```python
from build123d import *

# Parameters (mm, degrees)
SKETCH1_R           = 2.9718
SKETCH1_W           = 47.1424
SKETCH1_H           = 22.225
SKETCH1_R_2         = 2.4892
BOSS_EXTRUDE1_DEPTH = 3.175
SKETCH2_W           = 85.2424
SKETCH2_H           = 3.175
BOSS_EXTRUDE2_DEPTH = 3.175


with BuildPart() as part:
    # Sketch1 → Boss-Extrude1 (new body)
    with BuildSketch(Plane.XY):
        Polygon((37.4777, 9.5377), (24.7777, 9.5377), (-35.0647, 9.5377), (-47.7647, 9.5377), (-47.7647, -25.3873), (-35.0647, -25.3873), (12.0777, -25.3873), (24.7777, -25.3873), (37.4777, -25.3873), align=None)
        with Locations((-32.941818083, -7.9248)):
            Circle(SKETCH1_R, mode=Mode.SUBTRACT)
        with Locations((-5.1435, -7.9248)):
            Rectangle(SKETCH1_W, SKETCH1_H, mode=Mode.SUBTRACT)
        with Locations((23.471581917, -7.9248)):
            Circle(SKETCH1_R, mode=Mode.SUBTRACT)
        Polygon((37.4777, -41.2623), (37.4777, -25.3873), (24.7777, -25.3873), (12.0777, -25.3873), (12.0777, -41.2623), align=None)
        with Locations((23.471581917, -33.3248)):
            Circle(SKETCH1_R_2, mode=Mode.SUBTRACT)
    extrude(amount=BOSS_EXTRUDE1_DEPTH)

    # Sketch2 → Boss-Extrude2 (add)
    with BuildSketch(Plane(origin=(0, 0, 0), x_dir=(-1, 0, 0), z_dir=(0, 0, -1))):
        with Locations((5.1435, 7.9502)):
            Rectangle(SKETCH2_W, SKETCH2_H)
    extrude(amount=BOSS_EXTRUDE2_DEPTH)


solid = part.part
```
Geometry check sheet. Reference: the model listing, model coordinates, mm. A direction names the side the tool comes from. Give positions to 0.01 mm unless a question says otherwise; leave off trailing zeros. Order: outer loops, then holes, each group sorted by start corner. A loop starts at its lowest first (then second) coordinate and runs counter-clockwise, first axis right, second up. Notation, with made-up numbers: (-35, -35.75) -> (18, -35.75) arc R23 ccw to (18, -19.75) -> close; hole circle Ø1 at (48, 59). An arc over 180 degrees is marked (long way). Write each question's results on one line, items separated by ' | '. Start each with the question number.
(1) Sectioned sample at D-D (y = -7). Enter the section's corners in (x, z) (3 decimals).
(2) Scan lines: line 1 (X direction, y = -8, z = 2); line 2 (Y direction, x = 18, z = 2); line 3 (Y direction, x = -10, z = -1.5). Record each from-to range of solid material in increasing order.
(3) Access from +Z, -Z, +X, -X, +Y, -Y to the whole of each face (thin tool, end or side, straight path). Record for faces 4 (the face through (-18, -25.387, 2)), 5 (the face through (18.428, -8, 2)), 6 (the face through (4, -22, 0)).
(4) Sectioned sample at A-A (y = -16). Enter the section's corners in (x, z) (3 decimals).
(5) Mould release check, pull along Y, two halves, no side actions. Record for faces 1 (the face through (12.078, -33, 2)), 2 (the face through (25, -41.262, 2)), 3 (the face through (-5, 3.188, 2)): pulls with the +Y half, pulls with the -Y half, needs draft (parallel to the pull), parting line crosses it, or undercut.
(6) Sectioned sample at C-C (z = 2.25). Enter the section's corners in (x, y).
(7) Sectioned sample at B-B (x = 0). Enter the section's corners in (y, z) (3 decimals).
(8) Gauge pin test, flat ends, axial feed: P1, Ø6, axis at x = -26.5, y = -12.5, coming from the +Z side (3 decimals); P2, Ø1, axis at x = -13, z = 1.5, coming from the -Y side; P3, Ø8, axis at x = 23.47, y = -33.32, coming from the -Z side; P4, Ø1.6, axis at x = -18, z = -2, coming from the -Y side. Record the tip position at first contact, or that the pin passes through.
Answer below:
1) outline: (-47.765, 0) -> (-35.766, 0) -> (-35.766, 3.175) -> (-47.765, 3.175) -> close; (-30.118, 0) -> (-28.715, 0) -> (-28.715, 3.175) -> (-30.118, 3.175) -> close; (18.428, 0) -> (20.647, 0) -> (20.647, 3.175) -> (18.428, 3.175) -> close; (26.296, 0) -> (37.478, 0) -> (37.478, 3.175) -> (26.296, 3.175) -> close
2) line 1: -47.76 to -35.91, -29.97 to -28.71, 18.43 to 20.5, 26.44 to 37.48 | line 2: -41.26 to -19.04, 3.19 to 9.54 | line 3: 6.36 to 9.54
3) face 4: +Z, -Z, -X, -Y | face 5: +Z, -Z | face 6: -Z, +X, -X, -Y
4) outline: (-47.765, 0) -> (-28.715, 0) -> (-28.715, 3.175) -> (-47.765, 3.175) -> close; (18.428, 0) -> (37.478, 0) -> (37.478, 3.175) -> (18.428, 3.175) -> close
5) face 1: needs draft | face 2: pulls with the -Y half | face 3: undercut
6) outline: (-47.76, -25.39) -> (12.08, -25.39) -> (12.08, -41.26) -> (37.48, -41.26) -> (37.48, 9.54) -> (-47.76, 9.54) -> close; hole circle Ø5.94 at (-32.94, -7.92); hole (-28.71, -19.04) -> (18.43, -19.04) -> (18.43, 3.19) -> (-28.71, 3.19) -> close; hole circle Ø5.94 at (23.47, -7.92); hole circle Ø4.98 at (23.47, -33.32)
7) outline: (-25.387, 0) -> (-19.037, 0) -> (-19.037, 3.175) -> (-25.387, 3.175) -> close; (3.188, 0) -> (6.363, 0) -> (6.363, -3.175) -> (9.538, -3.175) -> (9.538, 3.175) -> (3.188, 3.175) -> close
8) P1: z = 3.175 | P2: y = -25.39 | P3: z = 0 | P4: y = 6.36
